Here's the drawing with two shaded views (mm, measured from the low corner). I have some questions. A direction names the side the tool comes from. Round coordinates to 2 decimals unless told otherwise and drop trailing zeros. Order: outer loops, then holes, each group sorted by start corner. A loop starts at its lowest first (then second) coordinate and runs counter-clockwise, first axis right, second up.
Q1. If we section it at C-C (y = 9): Please give me the cut outline in (x, z), plus the area to 3 significant figures.
Q2. If I drill on line 1 (Y direction, x = 25.5, z = 9.5); line 2 (X direction, y = 25, z = 1.5); line 3 (X direction, y = 4, z = 6.5), over which ranges is the centre line in solid material (lowest first)?
Q3. If we section it at B-B (x = 25): Please give me the cut outline in (y, z).
Q4. If we section it at A-A (z = 3.75): Please give me the cut outline in (x, y), plus the area to 3 significant figures.
Q5. For the marked faces 1 and 2, which set-ups out of +Z, -Z, +X, -X, +Y, -Y let a thin tool reach every point of the face, with its end or its side?
Q6. Will these pins go through, and if not, where does the flat tip stop? P1, Ø1.9, axis at x = 51.5, y = 28.5, coming from the -Z side; P2, Ø7, axis at y = 21.5, z = 12.5, coming from the +X side; P3, Ø0.5, axis at x = 47.5, z = 11.5, coming from the +Y side.
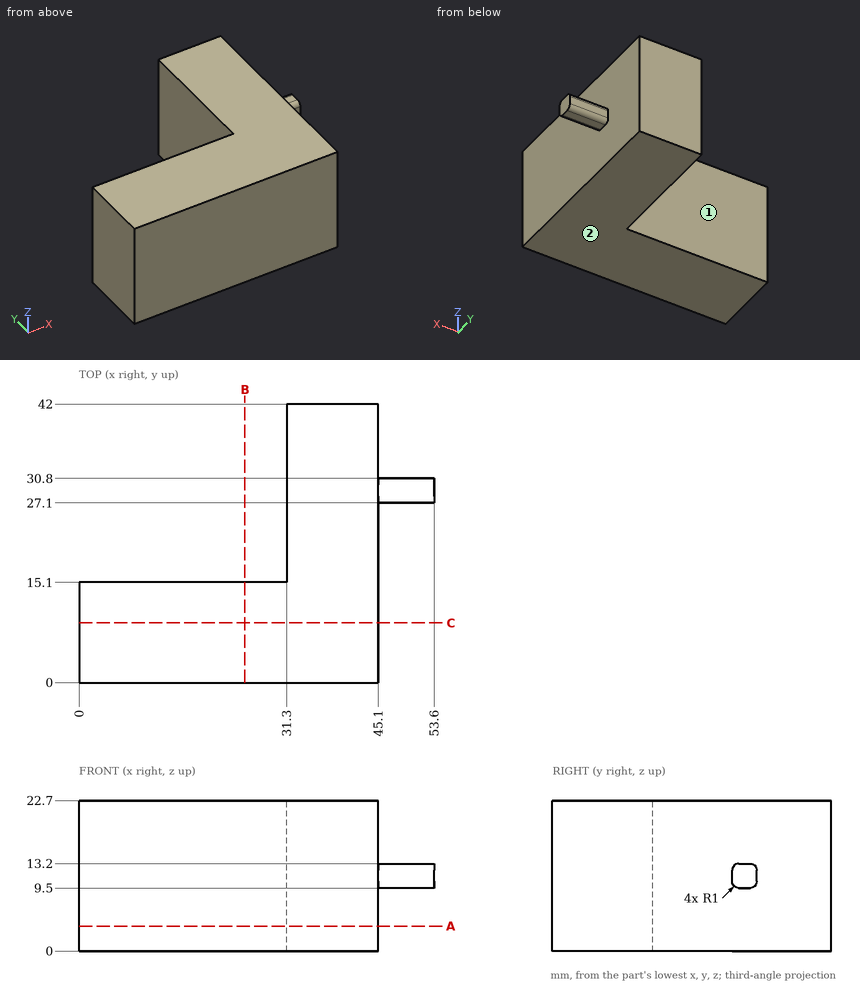
Solution:
1. outline: (0, 0) - (45.1, 0) - (45.1, 22.7) - (0, 22.7) - close
1. area: 1,020 mm2
2. line 1: y = 0 to 15.1
2. line 2: x = 31.3 to 45.1
2. line 3: x = 0 to 45.1
3. outline: (0, 0) - (15.1, 0) - (15.1, 22.7) - (0, 22.7) - close
4. outline: (0, 0) - (45.1, 0) - (45.1, 42) - (31.3, 42) - (31.3, 15.1) - (0, 15.1) - close
4. area: 1,050 mm2
5. face 1: +Z, -Z, -X, +Y
5. face 2: -Z, +X, -X, +Y, -Y
6. P1: stops at z = 9.5
6. P2: stops at x = 45.1
6. P3: stops at y = 30.8
